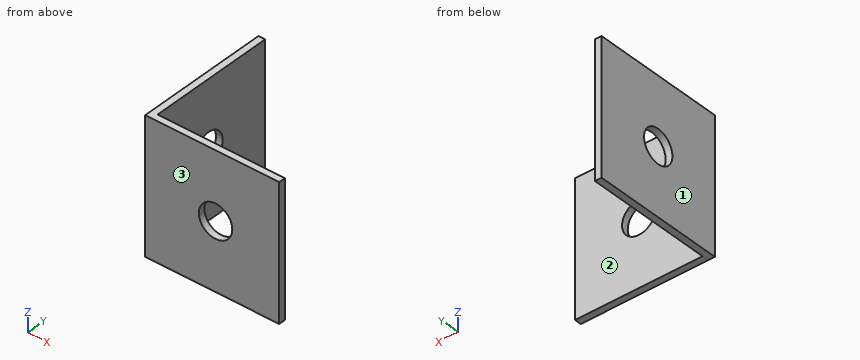
from build123d import *

# Parameters (mm, degrees)
SKETCH1_W           = 25.4
SKETCH1_H           = 25.4
BOSS_EXTRUDE1_DEPTH = 1.27
BOSS_EXTRUDE2_DEPTH = 1.27
SKETCH3_R           = 3.175
CUT_EXTRUDE1_DEPTH  = 1.27
SKETCH4_R           = 3.175
CUT_EXTRUDE2_DEPTH  = 1.27


with BuildPart() as part:
    # Sketch1 → Boss-Extrude1 (new body)
    with BuildSketch(Plane(origin=(0, 0, 0), x_dir=(0, 0, -1), z_dir=(1, 0, 0))):
        Rectangle(SKETCH1_W, SKETCH1_H)
    extrude(amount=BOSS_EXTRUDE1_DEPTH)

    # Sketch2 → Boss-Extrude2 (add)
    with BuildSketch(Plane.XZ.offset(12.7)):
        Polygon((1.27, 12.7), (25.4, 12.7), (25.4, -12.738650011), (1.27, -12.7), align=None)
    extrude(amount=-BOSS_EXTRUDE2_DEPTH)

    # Sketch3 → Cut-Extrude1 (cut)
    with BuildSketch(Plane(origin=(1.27, 0, 0), x_dir=(0, 0, -1), z_dir=(1, 0, 0))):
        Circle(SKETCH3_R)
    extrude(amount=-CUT_EXTRUDE1_DEPTH, mode=Mode.SUBTRACT)

    # Sketch4 → Cut-Extrude2 (cut)
    with BuildSketch(Plane(origin=(0, -11.43, 0), x_dir=(1, 0, 0), z_dir=(0, 1, 0))):
        with Locations(Location((13.335, 0.009662503, 0), (0, 0, 270))):
            Circle(SKETCH4_R)
    extrude(amount=-CUT_EXTRUDE2_DEPTH, mode=Mode.SUBTRACT)


solid = part.part
Can you work these out from the model? Positions are in its coordinate system, mm. Face numbers are marked on the shaded views. Round coordinates to 2 decimals unless told otherwise and drop trailing zeros. Write each loop counter-clockwise with the first axis right and the second up, starting at its lowest first coordinate (ties: lowest second). Pieces come first, ordered by that corner, then holes. Notation, with made-up numbers: (17.25, 52.25) -> (21.25, 52.25) arc R16 cw to (21.25, 69.25) -> close; hole circle Ø9 at (48, 60). An arc over 180 degrees is marked (long way). One line per question, with ' | ' between items. Start each with the question number.
1) Suppose I cut it at B-B on z = 0.5. Write out the boundary of the cut face in (x, y).
2) I'm going to push flat-ended pins straight in: P1, Ø3, axis at x = 4, y = 6.5, coming from the +Z side; P2, Ø10, axis at x = 10.5, z = 4.5, coming from the +Y side; P3, Ø1.4, axis at x = 0.5, y = -0.5, coming from the -Z side; P4, Ø4, axis at y = 2, z = -8, coming from the +X side. Where does each tip first touch, or does it pass through?
3) If we mould it in two halves opening along Y, with no side actions, what happens to the marked faces 1, 2 and 3? For each: released by +Y, released by -Y, zero draft, split by the parting line, or undercut.
4) Suppose I cut it at C-C on z = 9. Write out the boundary of the cut face in (x, y).
5) Suppose I cut it at A-A on y = 0. Write out the boundary of the cut face in (x, z) (3 decimals).
6) Suppose I cut it at D-D on y = -6. Write out the boundary of the cut face in (x, z).
7) I need wall thicknesses on line 1 (Y direction, x = 0.4, z = 0) (3 decimals); line 2 (Y direction, x = 1.5, z = 1.5); line 3 (X direction, y = -11, z = 6). Which ranges of each line are inside material? Lowest first, please. Write a range as [from, to].
Return value:
1) outline: (0, -12.7) -> (10.2, -12.7) -> (10.2, -11.43) -> (1.27, -11.43) -> (1.27, -3.14) -> (0, -3.14) -> close; (0, 3.14) -> (1.27, 3.14) -> (1.27, 12.7) -> (0, 12.7) -> close; (16.47, -12.7) -> (25.4, -12.7) -> (25.4, -11.43) -> (16.47, -11.43) -> close
2) P1: passes through | P2: stops at y = -11.43 | P3: stops at z = -12.7 | P4: stops at x = 1.27
3) face 1: zero draft | face 2: released by +Y | face 3: released by -Y
4) outline: (0, -12.7) -> (25.4, -12.7) -> (25.4, -11.43) -> (1.27, -11.43) -> (1.27, 12.7) -> (0, 12.7) -> close
5) outline: (0, -12.7) -> (1.27, -12.7) -> (1.27, -3.175) -> (0, -3.175) -> close; (0, 3.175) -> (1.27, 3.175) -> (1.27, 12.7) -> (0, 12.7) -> close
6) outline: (0, -12.7) -> (1.27, -12.7) -> (1.27, 12.7) -> (0, 12.7) -> close
7) line 1: y = [-12.7, -3.175], [3.175, 12.7] | line 2: y = [-12.7, -11.43] | line 3: x = [0, 1.27]
